Input: dimensioned drawing with shaded views. Units: mm. Origin: part minimum x, y, z. A direction names the side the tool comes from. Round coordinates to 2 decimals unless told otherwise and drop trailing zeros. Write each loop counter-clockwise with the first axis right and the second up, starting at its lowest first coordinate (ties: lowest second). Pieces come first, ordered by that corner, then holes. Notation, with made-up numbers: (58, 30.25) - (91, 30.25) arc R29 cw to (91, 56.25) - close; hole circle Ø4 at (88.5, 25.5). An arc over 180 degrees is marked (long way). Write item = value, one per line. Start each with the question number.
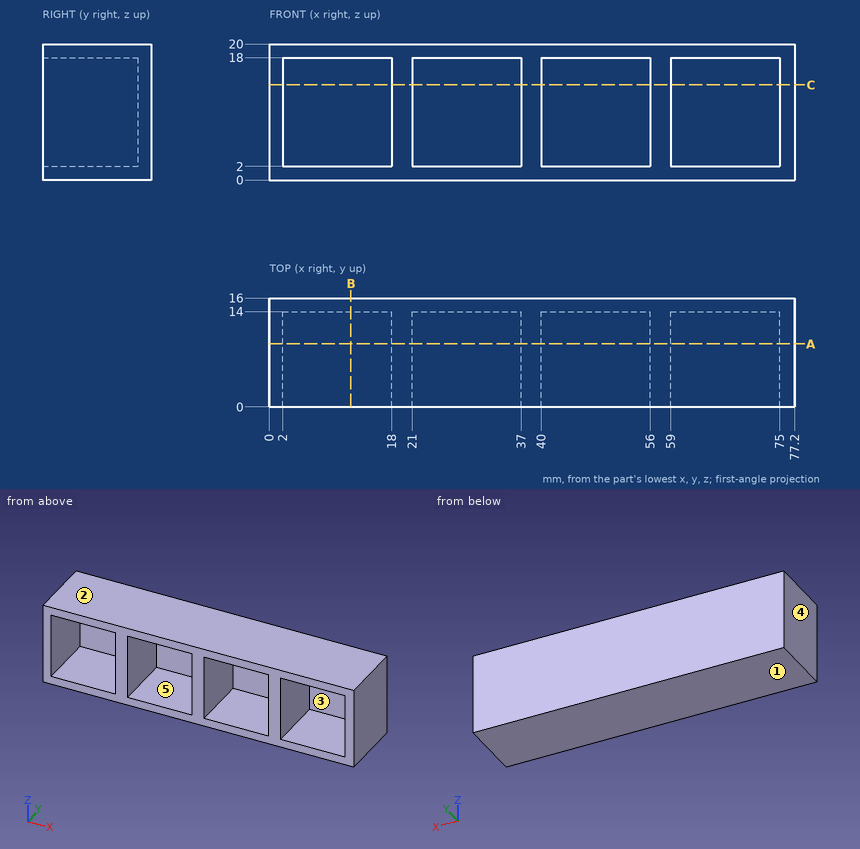
(1) Reachability of the marked faces 4 and 5 from +Z, -Z, +X, -X, +Y, -Y: full face, straight path, thin tool, end or side. Return the list, or none.
(2) Section C-C (z = 14). Return the cut outline in (x, y), plus the area to 3 significant figures.
(3) Contact query for flat-ended pins moving along their axis: P1, Ø2, axis at x = 28, y = 13.5, coming from the -Z side; P2, Ø1.5, axis at x = 29.5, z = 7, coming from the -Y side. Output: stop coordinate, or through.
(4) Section B-B (x = 12). Return the cut outline in (y, z).
(5) Section A-A (y = 9.25). Return the cut outline in (x, z).
(6) Ray query, L1, parallel to X at y = 2.5, z = 5.75; L2, parallel to Z at x = 69, y = 1.5; L3, parallel to Y at x = 34, z = 17. Return the intervals inside material, ascending. Write a range as from..to.
(7) Pull-direction query (Z, two-part tool) for the marked faces 1, 2 and 3; classes: +Z half, -Z half, draft (parallel to the pull), parting line (faces both ways), or undercut.
Solution:
q1.face_4 = +Z, -Z, -X, +Y, -Y
q1.face_5 = -Y
q2.outline = (0, 0) - (2, 0) - (2, 14) - (18, 14) - (18, 0) - (21, 0) - (21, 14) - (37, 14) - (37, 0) - (40, 0) - (40, 14) - (56, 14) - (56, 0) - (59, 0) - (59, 14) - (75, 14) - (75, 0) - (77.2, 0) - (77.2, 16) - (0, 16) - close
q2.area = 339 mm^2
q3.P1 = 0
q3.P2 = 14
q4.outline = (0, 0) - (16, 0) - (16, 20) - (0, 20) - (0, 18) - (14, 18) - (14, 2) - (0, 2) - close
q5.outline = (0, 0) - (77.2, 0) - (77.2, 20) - (0, 20) - close; hole (2, 2) - (18, 2) - (18, 18) - (2, 18) - close; hole (21, 2) - (37, 2) - (37, 18) - (21, 18) - close; hole (40, 2) - (56, 2) - (56, 18) - (40, 18) - close; hole (59, 2) - (75, 2) - (75, 18) - (59, 18) - close
q6.L1 = 0..2, 18..21, 37..40, 56..59, 75..77.2
q6.L2 = 0..2, 18..20
q6.L3 = 14..16
q7.face_1 = -Z half
q7.face_2 = +Z half
q7.face_3 = undercut
